from build123d import *

# Parameters (mm, degrees)
SKETCH1_R             = 33.147
BOSS_EXTRUDE1_DEPTH   = 2.9718
F_8_CLEARANCE_HOLE1_D = 4.3053
FILLET1_R             = 2.54


with BuildPart() as part:
    # Sketch1 → Boss-Extrude1 (new body)
    with BuildSketch(Plane(origin=(0, 0, 0), x_dir=(1, 0, 0), z_dir=(0, 1, 0))):
        Polygon((720.939652548, 26.242162499), (720.939652548, -113.457837501), (746.339652548, -113.457837501), (746.339652548, -132.507837501), (1355.939652548, -132.507837501), (1355.939652548, 45.292162499), (746.339652548, 45.292162499), (746.339652548, 26.242162499), align=None)
        with Locations(Location((1299.335652548, -43.607837501, 0), (0, 0, 270))):
            Circle(SKETCH1_R, mode=Mode.SUBTRACT)
        with Locations(Location((1198.753990482, -46.877734612, 0), (0, 0, 270))):
            Circle(SKETCH1_R, mode=Mode.SUBTRACT)
        with Locations(Location((1098.172328416, -50.147631723, 0), (0, 0, 270))):
            Circle(SKETCH1_R, mode=Mode.SUBTRACT)
        with Locations(Location((997.59066635, -53.417528834, 0), (0, 0, 270))):
            Circle(SKETCH1_R, mode=Mode.SUBTRACT)
        with Locations(Location((897.009004284, -56.687425945, 0), (0, 0, 270))):
            Circle(SKETCH1_R, mode=Mode.SUBTRACT)
        with Locations(Location((796.427342219, -59.957323056, 0), (0, 0, 270))):
            Circle(SKETCH1_R, mode=Mode.SUBTRACT)
    extrude(amount=BOSS_EXTRUDE1_DEPTH)

    # #8 Clearance Hole1 (through all)
    with Locations(Plane(origin=(0, 2.9718, 0), x_dir=(1, 0, 0), z_dir=(0, 1, 0))):
        with Locations((759.039652548, 38.942162499), (759.039652548, -126.157837501), (953.772985881, -126.157837501), (953.772985881, 38.942162499), (1148.506319214, 38.942162499), (1148.506319214, -126.157837501), (1343.239652548, -126.157837501), (1343.239652548, 38.942162499), (1249.018252548, -43.607837501), (1051.139652548, -43.607837501), (846.479052548, -43.607837501)):
            Hole(F_8_CLEARANCE_HOLE1_D / 2)

    # Fillet1
    fillet1_edges = [part.edges().sort_by_distance(p)[0] for p in [
        (746.339652548, 1.4859, 132.507837501),
        (720.939652548, 1.4859, 113.457837501),
        (720.939652548, 1.4859, -26.242162499),
        (746.339652548, 1.4859, -45.292162499),
        (1355.939652548, 1.4859, -45.292162499),
        (1355.939652548, 1.4859, 132.507837501),
    ]]
    fillet(fillet1_edges, radius=FILLET1_R)


solid = part.part
For this review, take the finished solid that the model builds, in its own axes (mm). Round coordinates to 2 decimals unless told otherwise and drop trailing zeros. Order: outer loops, then holes, each group sorted by start corner. A loop starts at its lowest first (then second) coordinate and runs counter-clockwise, first axis right, second up. Notation, with made-up numbers: M 77,-6.5 L 95,-6.5 A30 ccw 95,18.5 Z; hole C -26.75,9 d2. An arc over 180 degrees is marked long. Write each question's results on one line, items separated by ' | '. Start each with the question number.
1. Clearance check with flat-ended pins moving along their axes: pin 1 Ø0.9 at (y, z) = (2, 125) entering from -X; pin 2 Ø1.5 at (x, y) = (739, 2) entering from +Z. State where each tip first meets the part, or that it passes through.
2. Draft analysis for pull direction Z (two halves, no side actions). For faces 1 (the face through (1034, 0, 42)), 2 (the face through (1221.16, 1.47, 22.45)), 3 (the face through (1030.456, 1.465, 49.102)), state which applies: pulls with the +Z half, pulls with the -Z half, needs draft (parallel to the pull), parting line crosses it, or undercut.
3. Add section C-C (y = 0.65). State how many separate pieces and enclosed holes the cut face has, then the cut area to 3 significant figures.
4. Add section B-B (x = 888.5). State the section outline as (y, z) points.
5. To check wall thickness, follow L1, parallel to Z at x = 797, y = 2.8; L2, parallel to X at y = 0.65, z = 20; L3, parallel to Z at x = 911.5, y = 1.75. State the ranges of each line that lie inside material, in increasing order. Write a range as [from, to].
6. Add section A-A (z = 52). State the section outline as (x, y) points, then the cut area to 3 significant figures.
Output values:
1) pin 1: x = 746.34 | pin 2: z = 113.46
2) face 1: needs draft | face 2: undercut | face 3: undercut
3) separate pieces: 1 | enclosed holes: 17 | area: 91,100 mm^2
4) outline: M 0,-45.29 L 2.97,-45.29 L 2.97,24.65 L 0,24.65 Z; M 0,88.72 L 2.97,88.72 L 2.97,132.51 L 0,132.51 Z
5) L1: [-45.29, 26.82], [93.1, 132.51] | L2: [720.94, 1084.39], [1111.95, 1179.36], [1218.15, 1276.07], [1322.6, 1355.94] | L3: [-45.29, 26.88], [86.5, 132.51]
6) outline: M 720.94,0 L 764.25,0 L 764.25,2.97 L 720.94,2.97 Z; M 828.61,0 L 864.2,0 L 864.2,2.97 L 828.61,2.97 Z; M 929.82,0 L 964.47,0 L 964.47,2.97 L 929.82,2.97 Z; M 1030.71,0 L 1065.08,0 L 1065.08,2.97 L 1030.71,2.97 Z; M 1131.27,0 L 1166.01,0 L 1166.01,2.97 L 1131.27,2.97 Z; M 1231.5,0 L 1267.27,0 L 1267.27,2.97 L 1231.5,2.97 Z; M 1331.4,0 L 1355.94,0 L 1355.94,2.97 L 1331.4,2.97 Z | area: 722 mm^2
